For this review, take the finished solid that the model builds, in its own axes (mm). A direction names the side the tool comes from. Give positions to 0.01 mm unless a question says otherwise; leave off trailing zeros. Write each loop counter-clockwise with the first axis right and the second up, starting at its lowest first coordinate (ties: lowest second). Pieces come first, ordered by that corner, then holes. Notation, with made-up numbers: M 52,53.5 L 83,53.5 A18 ccw 83,79.5 Z; hole C 4.5,-36 d7. An arc over 180 degrees is marked long. Use one line per item in the form item = value. Start each with the question number.
Q1. Tool access review of faces 5 (the flat face through (1, 42, -1)), 6 (the flat face through (0, 83, -4)): name each direction out of +Z, -Z, +X, -X, +Y, -Y from which nothing blocks a thin tool from reaching the whole face with its end or side.
Q2. Consider section D-D on y = 6. Write out the cut boundary in (x, z).
Q3. Mouldability with a two-part tool opening along X and no side actions: class faces 1 (the flat face through (0, 33, -8)), 2 (the cylindrical face through (3.96, 41.56, -3.94)), 3 (the cylindrical face through (-5.04, 34.56, -3.94)), 4 (the flat face through (-8, 41, -4)) as released by +X, released by -X, zero draft, split by the parting line, or undercut.
Q4. Consider section A-A on y = 51. Write out the cut boundary in (x, z), and give its area (3 significant figures).
Q5. Consider section B-B on z = -7. Give the number of separate pieces and of enclosed holes in the cut face, and give its area (3 significant figures).
Q6. For probe 1 along X at (y, z) = (68.5, -1.75); probe 2 along X at (y, z) = (51.5, -4.25); probe 3 along Z at (x, y) = (-0.25, 5), list the stretches that pass through material, from the lowest coordinate up. Write a range as [from, to].
Autodesk Fusion 360 part; units mm, degrees
sketch "tree" plane through (0, 0, 0) normal (0, 0, 1) x (1, 0, 0)
  line L0 (0, 0) -> (0, 94.3715) construction
  circle A0 centre (-4.5, 30) radius 2.5
  circle A1 centre (4.5, 30) radius 2.5
  circle A2 centre (-4.5, 37) radius 2.5
  circle A3 centre (4.5, 37) radius 2.5
  circle A4 centre (-4.5, 44) radius 2.5
  circle A5 centre (4.5, 44) radius 2.5
  circle A6 centre (-4.5, 51) radius 2.5
  circle A7 centre (4.5, 51) radius 2.5
  circle A8 centre (-4.5, 58) radius 2.5
  circle A9 centre (4.5, 58) radius 2.5
  circle A10 centre (-4.5, 65) radius 2.5
  circle A11 centre (4.5, 65) radius 2.5
  circle A12 centre (-4.5, 72) radius 2.5
  circle A13 centre (4.5, 72) radius 2.5
  circle A14 centre (-4.5, 79) radius 2.5
  circle A15 centre (4.5, 79) radius 2.5
  line L1 (-1, 83) -> (1, 83)
  line L2 (1, 83) -> (1, 0)
  line L3 (1, 0) -> (-1, 0)
  line L4 (-1, 0) -> (-1, 83)
  dimension "d7" = 5
  dimension "d10" = 9
  dimension "d11" = 7
  dimension "d12" = 2
  dimension "d13" = 30
  dimension "d14" = 4
sketch "plate" plane through (0, 0, 0) normal (0, 0, 1) x (1, 0, 0)
  line L0 (-8, 83) -> (8, 83)
  line L1 (8, 83) -> (8, 0)
  line L2 (8, 0) -> (-8, 0)
  line L3 (-8, 0) -> (-8, 83)
  line L4 (0, 0) -> (0, 94.3715)
  point P0 (1, 83)
  dimension "d16" = 8
extrude "Extrude1" add sketch "plate" against normal blind 8
extrude "Extrude2" cut sketch "tree" against normal through all contours A0 | A1 | A2 | A3 | A4 | A5 | A6 | A7 | A8 | A9 | A10 | A11 | A12 | A13 | A14 | A15
extrude "Extrude3" cut sketch "tree" against normal blind 2 contours L1 L2 L3 L4
equation "led_dia = 5 mm"
equation "wire_dia = 2 mm"
equation "led_vspace = 2 mm"
equation "led_hspace = 2 mm"
equation "wire_bottom_stickout = 30 mm"
equation "wire_top_stickout = 4 mm"
equation "d7 = led_dia"
equation "d10 = led_dia + led_hspace + wire_dia"
equation "d11 = led_dia + led_vspace"
equation "d12 = wire_dia"
equation "d13 = wire_bottom_stickout"
equation "d14 = wire_top_stickout"
equation "d16 = led_dia + led_hspace + 1 mm"
Working result:
q1.face_5 = +Z, +Y, -Y
q1.face_6 = +Z, -Z, +X, -X, +Y
q2.outline = M -8,-8 L 8,-8 L 8,0 L 1,0 L 1,-2 L -1,-2 L -1,0 L -8,0 Z
q3.face_1 = zero draft
q3.face_2 = undercut
q3.face_3 = undercut
q3.face_4 = released by -X
q4.outline = M -8,-8 L -7,-8 L -7,0 L -8,0 Z; M -2,-8 L 2,-8 L 2,0 L 1,0 L 1,-2 L -1,-2 L -1,0 L -2,0 Z; M 7,-8 L 8,-8 L 8,0 L 7,0 Z
q4.area = 44.0 mm²
q5.separate_pieces = 1
q5.enclosed_holes = 16
q5.area = 1,010 mm²
q6.probe_1 = [-8, -1], [1, 8]
q6.probe_2 = [-8, -6.95], [-2.05, 2.05], [6.95, 8]
q6.probe_3 = [-8, -2]
